```python
from build123d import *


with BuildPart() as part:
    # Sketch1 → Revolve1 (revolve)
    with BuildSketch(Plane.XY, mode=Mode.PRIVATE) as revolve1_sk:
        with BuildLine():
            Line((0, 0), (0, -72.5))
            Line((0, -72.5), (5, -72.5))
            Line((5, -72.5), (5, -30))
            Line((5, -30), (9, -30))
            Line((9, -30), (9, -27))
            Line((9, -27), (14.25, -27))
            Line((14.25, -27), (14.25, -24))
            Line((14.25, -24), (13.25, -24))
            add(Edge.make_bspline(
                [(13.25, -24), (12.876288893, -20.234768096), (12.502577786, -16.469536192), (12.12886668, -12.704304288), (12.10802883, -12.494357794), (12.06635313, -12.074464806), (12.003839581, -11.444625323), (11.962163881, -11.024732334), (11.941326032, -10.81478584), (11.913600396, -10.535443194), (11.858149124, -9.976757903), (11.666555139, -9.148985732), (11.514124842, -8.608285073), (11.428528654, -8.340938262), (9.779050122, -3.189040311), (5.409513095, 0), (0, 0)],
                knots=[0, 0, 0, 0, 0.379321245, 0.379321245, 0.379321245, 0.400471912, 0.421622579, 0.442773246, 0.442773246, 0.442773246, 0.470915098, 0.499056951, 0.527198803, 0.527198803, 0.527198803, 1, 1, 1, 1], degree=3, weights=[1, 1, 1, 1, 1, 1, 1, 1, 1, 1, 1, 1, 1, 1, 0.871833681, 0.871833681, 1]))
        make_face()
    revolve(revolve1_sk.sketch.rotate(Axis((0, 0, 0), (0, -1, 0)), 180), axis=Axis((0, 0, 0), (0, -1, 0)))


solid = part.part
```
Geometry: final body of the model. Coordinates: model frame, mm. A direction names the side the tool comes from. Coordinates: 2 decimals unless noted, no trailing zeros. Loops run counter-clockwise (first coordinate to the right, second up) from the corner with the lowest first, then second, coordinate; pieces in that order, holes last. Notation, with made-up numbers: (-38, -8) -> (-34, -8) arc R26 ccw to (-34, 15) -> close; hole circle Ø2 at (31.5, 74). An arc over 180 degrees is marked (long way). Use a Markdown table: item, result. Add a question column.
(1) Section query A-A, the plane y = -41. Return loops of the section in (x, z).
(2) Access query for faces 1 (the flat face through (0, -72.5, 0)), 2 (the flat face through (-4, -24, 13)), 3 (the cylindrical face through (5, -51, 0)). Directions: +Z, -Z, +X, -X, +Y, -Y. A direction counts if a zero-diameter tool reaches every point of the face in a straight line with its end or side. Return the directions, or none.
(3) Line query: line 1 along Y through (x, z) = (8, -11.25); line 2 along Z through (x, y) = (-4.5, -7.5); line 3 along Z through (x, y) = (4.5, -3.5). Output: solid intervals per line, ascending.
(4) Pin query (flat end, axial travel): pin 1 Ø1.5 at (y, z) = (-7.5, -7) entering from +X; pin 2 Ø6 at (x, y) = (5.5, -8.5) entering from +Z; pin 3 Ø12 at (x, y) = (-1.5, -10) entering from +Z. Return the tip coordinate at first contact, or that it passes through.
Answer:
| question | item | result |
|---|---|---|
| 1 | outline | circle Ø10 at (0, 0) |
| 2 | face 1 | +Z, -Z, +X, -X, -Y |
| 2 | face 2 | +Y |
| 2 | face 3 | -Y |
| 3 | line 1 | y = -27 to -24 |
| 3 | line 2 | z = -10.17 to 10.17 |
| 3 | line 3 | z = -7.18 to 7.18 |
| 4 | pin 1 | stops at x = 9.31 |
| 4 | pin 2 | stops at z = 11.48 |
| 4 | pin 3 | stops at z = 12.44 |
